Design review of the part built by this model. Coordinates are the model's own, in mm. Round coordinates to 2 decimals unless told otherwise and drop trailing zeros. Order: outer loops, then holes, each group sorted by start corner. A loop starts at its lowest first (then second) coordinate and runs counter-clockwise, first axis right, second up. Notation, with made-up numbers: M 15.25,36.5 L 52.25,36.5 A20 cw 52.25,45.5 Z; hole C 69.5,-2.5 d8. An arc over 180 degrees is marked long. Write item = value, one per line. Start each with the question number.
```python
from build123d import *

# Parameters (mm, degrees)
SKETCH2_W               = 304.8
SKETCH2_H               = 304.8
BOSS_EXTRUDE1_DEPTH     = 12.7
SKETCH3_R               = 3.175
CUT_EXTRUDE1_DEPTH      = 343.16151121
SKETCH4_R               = 3.175
CUT_EXTRUDE2_DEPTH      = 358.845553564
CUT_EXTRUDE3_DEPTH      = 343.16151121
CUT_EXTRUDE3_DEPTH_BACK = 343.16151121
SKETCH8_R               = 3.089580747
SCALE1_SCALE            = 1.5


with BuildPart() as part:
    # Sketch2 → Boss-Extrude1 (new body)
    with BuildSketch(Plane(origin=(0, 0, 0), x_dir=(1, 0, 0), z_dir=(0, 1, 0))):
        with Locations((-98.440191388, 2.55215311)):
            Rectangle(SKETCH2_W, SKETCH2_H)
    extrude(amount=BOSS_EXTRUDE1_DEPTH)

    # Sketch3 → Cut-Extrude1 (cut, through all)
    with BuildSketch(Plane(origin=(53.959808612, 0, 0), x_dir=(0, 0, -1), z_dir=(1, 0, 0))):
        with Locations((2.55215311, 6.35)):
            Circle(SKETCH3_R)
    extrude(amount=-CUT_EXTRUDE1_DEPTH, mode=Mode.SUBTRACT)

    # Sketch4 → Cut-Extrude2 (cut, through all)
    with BuildSketch(Plane(origin=(-250.840191388, 0, 32.101609765), x_dir=(0, 0, 1), z_dir=(-1, 0, 0))):
        with Locations((-97.607511841, 7.050929825)):
            Circle(SKETCH4_R)
    extrude(amount=-CUT_EXTRUDE2_DEPTH, mode=Mode.SUBTRACT)

    # Sketch8 → Cut-Extrude3 (cut, two sides: drawn at the far end of the back side and taken through both)
    with BuildSketch(Plane.ZY.offset(250.840191388).offset(-CUT_EXTRUDE3_DEPTH_BACK)):
        with Locations((-85.030883776, 7.028633546)):
            Circle(SKETCH8_R)
    extrude(amount=CUT_EXTRUDE3_DEPTH + CUT_EXTRUDE3_DEPTH_BACK, mode=Mode.SUBTRACT)


with BuildPart() as part_1:
    # Scale1: scaled about (-98.440191388, 6.338736644, -1.369646506)
    add(part.part.scale(SCALE1_SCALE).moved(Location((49.220095694, -3.169368322, 0.684823253))))


solid = part_1.part
```
(1) Consider section A-A, the plane x = 93. Write out the cut boundary in (y, z) (1 decimal).
(2) For line 1 along Z through (x, y) = (-114.5, 10); line 2 along Z through (x, y) = (63, 8); line 3 along Z through (x, y) = (-272.5, 2), list the stretches that pass through material, from the lowest coordinate up. Write a range as [from, to].
(3) Insertion check: pin 1 (8 mm diameter, centred on y = 9, z = 0, fed in from +X); pin 2 (5.5 mm diameter, centred on y = 6.36, z = -3.14, fed in from -X). Each pin has a flat end and moves straight along its axis. Give the tip position at first contact, or say it passes through.
(4) Draft analysis for pull direction Z (two halves, no side actions). For faces 1 (the face through (-102, 6, -231.743)), 2 (the face through (-102, 6, 225.457)), 3 (the face through (130.16, 2, 0)), state which applies: pulls with the +Z half, pulls with the -Z half, needs draft (parallel to the pull), parting line crosses it, or undercut.
Completed:
q1.outline = M -3.2,-231.7 L 15.9,-231.7 L 15.9,225.5 L -3.2,225.5 Z; hole C 6.4,-3.1 d9.5; hole C 7.4,-97.6 d9.5; hole C 7.4,-126.9 d9.3
q2.line_1 = [-231.74, -130.68], [-123.04, -101.57], [-93.58, -6.21], [-0.08, 225.46]
q2.line_2 = [-231.74, -131.45], [-122.27, -102.3], [-92.85, -7.61], [1.33, 225.46]
q2.line_3 = [-231.74, -5.07], [-1.22, 225.46]
q3.pin_1 = 130.16
q3.pin_2 = through
q4.face_1 = pulls with the -Z half
q4.face_2 = pulls with the +Z half
q4.face_3 = needs draft
